```python
from build123d import *

# Parameters (mm, degrees)
SALIENTE_EXTRUIR1_DEPTH = 0.1


with BuildPart() as part:
    # Model → Saliente-Extruir1 (new body)
    with BuildSketch(Plane.XY):
        with BuildLine():
            ThreePointArc((22.540248989, 13.854945853), (26.36224915, 12.09625195), (30.548359243, 11.675334187))
            ThreePointArc((30.548359243, 11.675334187), (30.487312629, 12.373336734), (30.5695137, 13.069165182))
            ThreePointArc((30.5695137, 13.069165182), (31.081390856, 13.736758239), (31.921654238, 13.777454212))
            ThreePointArc((31.921654238, 13.777454212), (33.309090368, 13.333130187), (34.7477202, 13.103462905))
            ThreePointArc((34.7477202, 13.103462905), (35.76012095, 13.732496208), (35.451331706, 14.883707473))
            ThreePointArc((35.451331706, 14.883707473), (34.302777703, 15.641386071), (33.040248989, 16.188445853))
            ThreePointArc((33.040248989, 16.188445853), (34.617609881, 15.988093646), (36.188952789, 16.231177692))
            ThreePointArc((36.188952789, 16.231177692), (36.899751011, 17.188445853), (36.188952789, 18.145714014))
            ThreePointArc((36.188952789, 18.145714014), (34.888660423, 18.378666365), (33.569660753, 18.306092912))
            ThreePointArc((33.569660753, 18.306092912), (34.755020368, 18.932581608), (35.621884252, 19.955378023))
            ThreePointArc((35.621884252, 19.955378023), (35.642787011, 20.89656979), (34.872667415, 21.438044328))
            ThreePointArc((34.872667415, 21.438044328), (32.337672311, 21.27261115), (30.040248989, 20.188445853))
            ThreePointArc((30.040248989, 20.188445853), (24.906113256, 18.660760825), (22.540248989, 13.854945853))
        make_face()
    extrude(amount=SALIENTE_EXTRUIR1_DEPTH)


solid = part.part
```
Work out the finished part from the listing and answer in its coordinate system (mm). Give positions to 0.01 mm unless a question says otherwise; leave off trailing zeros. Order: outer loops, then holes, each group sorted by start corner. A loop starts at its lowest first (then second) coordinate and runs counter-clockwise, first axis right, second up. Notation, with made-up numbers: (83, 82) - (118, 82) arc R20 cw to (118, 106) - close; hole circle Ø3 at (-31.75, 87.25). An arc over 180 degrees is marked (long way). One line per item, written item: value. Start each with the question number.
1. Section A-A, the plane z = 0.05 is taken. Write down the section's boundary in (x, y).
2. Section B-B, the plane y = 18.75 is taken. Write down the section's boundary in (x, z), then the cut area to 3 significant figures.
3. Section C-C, the plane x = 26 is taken. Write down the section's boundary in (y, z).
4. Consider line 1 (Y direction, x = 34.25, z = 0.05); line 2 (Y direction, x = 30.75, z = 0.05); line 3 (Y direction, x = 24.5, z = 0.05). Determine where each line is inside the solid, lowest interval first.
Filled sheet:
1. outline: (22.54, 13.85) arc R12.77 ccw to (30.55, 11.68) arc R3.43 cw to (30.57, 13.07) arc R1 cw to (31.92, 13.78) arc R9.62 ccw to (34.75, 13.1) arc R1 ccw to (35.45, 14.88) arc R7.91 ccw to (33.04, 16.19) arc R5.7 ccw to (36.19, 16.23) arc R1 ccw to (36.19, 18.15) arc R5.7 ccw to (33.57, 18.31) arc R3.54 ccw to (35.62, 19.96) arc R1 ccw to (34.87, 21.44) arc R6.8 ccw to (30.04, 20.19) arc R6.69 ccw to start
2. outline: (25.01, 0) - (34.51, 0) - (34.51, 0.1) - (25.01, 0.1) - close
2. area: 0.949 mm²
3. outline: (12.2, 0) - (19.41, 0) - (19.41, 0.1) - (12.2, 0.1) - close
4. line 1: 13.16 to 15.67, 15.99 to 18.38, 18.59 to 21.49
4. line 2: 13.46 to 20.64
4. line 3: 12.76 to 18.29
